```python
from build123d import *


with BuildPart() as part:
    # Sketch1 → Revolve1 (revolve)
    with BuildSketch(Plane.XY, mode=Mode.PRIVATE) as revolve1_sk:
        with BuildLine():
            Line((-122, 4), (-122, 0))
            Line((-122, 0), (122, 0))
            Line((122, 0), (122, 4))
            Line((122, 4), (114, 4))
            Line((114, 4), (114, 3.5))
            ThreePointArc((114, 3.5), (113.5, 3), (113, 3.5))
            Line((113, 3.5), (113, 6))
            Line((113, 6), (100, 6))
            Line((100, 6), (100, 11.5))
            Line((100, 11.5), (98, 11.5))
            Line((98, 11.5), (98, 10))
            Line((98, 10), (-98, 10))
            Line((-98, 10), (-98, 11.5))
            Line((-98, 11.5), (-100, 11.5))
            Line((-100, 11.5), (-100, 6))
            Line((-100, 6), (-113, 6))
            Line((-113, 6), (-113, 3.5))
            ThreePointArc((-113, 3.5), (-113.5, 3), (-114, 3.5))
            Line((-114, 3.5), (-114, 4))
            Line((-114, 4), (-122, 4))
        make_face()
    revolve(revolve1_sk.sketch.rotate(Axis((-122, 0, 0), (1, 0, 0)), 270), axis=Axis((-122, 0, 0), (1, 0, 0)))


solid = part.part
```
Build history of the part. All positions in model axes, mm. A direction names the side the tool comes from. Give positions to 0.01 mm unless a question says otherwise; leave off trailing zeros. Loops run counter-clockwise (first coordinate to the right, second up) from the corner with the lowest first, then second, coordinate; pieces in that order, holes last.
1) Probe line 1 along X through (y, z) = (1.75, -10); line 2 along X through (y, z) = (1.5, -8.5); line 3 along Y through (x, z) = (75, 0.5). List the from-to ranges inside material, lowest first.
Values follow:
line 1: x = -100 to -98, 98 to 100
line 2: x = -100 to 100
line 3: y = -9.99 to 9.99
2) Two-plate mould, pull along X, no slides. Class faces 6 (the face through (106.409, 1.802, -5.723)), 7 (the face through (122, 0, 0)), 8 (the face through (-98, 5, -9)): released by +X, released by -X, zero draft, split by the parting line, or undercut.
Values follow:
face 6: zero draft
face 7: released by +X
face 8: undercut
3) Band-saw the part on B-B on x = 63. List the corners of the cut face in (y, z), then the cut area to 3 significant figures.
Values follow:
outline: circle Ø20 at (0, 0)
area: 314 mm2
4) Drop flat-ended pins along their axis: P1, Ø8, axis at y = -3, z = 9, coming from the +X side; P2, Ø4, axis at x = 38.5, z = 8.5, coming from the -Y side; P3, Ø10, axis at x = -68, z = -8, coming from the -Y side; P4, Ø11.5, axis at y = -1, z = 4, coming from the +X side. Give the stop position or say it passes through.
Values follow:
P1: stops at x = 113
P2: stops at y = -7.6
P3: stops at y = -9.54
P4: stops at x = 122
5) 3-axis set-ups, long thin cutter, end or side, ignore diameter. For faces 1 (the face through (-118.056, -3.905, 0.867)), 2 (the face through (-99.01, 9.7, -6.18)), 3 (the face through (-122, 0, 0)), 4 (the face through (-113, -3, -3)), 5 (the face through (100, -5, 5)): which of +Z, -Z, +X, -X, +Y, -Y reach the whole face in a straight line?
Values follow:
face 1: -X
face 2: +X, -X
face 3: +Z, -Z, -X, +Y, -Y
face 4: none
face 5: +X
6) Band-saw the part on A-A on z = 8. List the corners of the cut face in (x, y).
Values follow:
outline: (-100, -8.26) - (-98, -8.26) - (-98, -6) - (98, -6) - (98, -8.26) - (100, -8.26) - (100, 8.26) - (98, 8.26) - (98, 6) - (-98, 6) - (-98, 8.26) - (-100, 8.26) - close
